The drawing under review shows one solid part. Ordinate dimensions are in mm from its lowest x, y, z. Give positions to 0.01 mm unless a question says otherwise; leave off trailing zeros. Write each loop counter-clockwise with the first axis right and the second up, starting at its lowest first coordinate (ties: lowest second). Pieces come first, ordered by that corner, then holes.
Q1. We need section C-C (x = 4). Write out the cut boundary in (y, z).
Q2. Insertion check: P1, Ø1.7, axis at x = 36.5, z = 17, coming from the +Y side; P2, Ø1.8, axis at y = 2.5, z = 26, coming from the +X side. Each pin has a flat end and moves straight along its axis. Give the tip position at first contact, or say it passes through.
Q3. We need section B-B (z = 4). Write out the cut boundary in (x, y), then the cut area to 3 significant figures.
Q4. We need section D-D (y = 2.5). Give the number of separate pieces and of enclosed holes in the cut face, then the cut area to 3 significant figures.
Q5. For line 1 (X direction, y = 2.05, z = 4); line 2 (Z direction, x = 20.5, y = 4.4); line 3 (X direction, y = 0.55, z = 30.5), list the stretches that pass through material, from the lowest coordinate up.
Q6. We need section A-A (x = 26). Write out the cut boundary in (y, z).
Q7. Mouldability with a two-part tool opening along Z and no side actions: class the marked faces 1, 2 and 3 as released by +Z, released by -Z, zero draft, split by the parting line, or undercut.
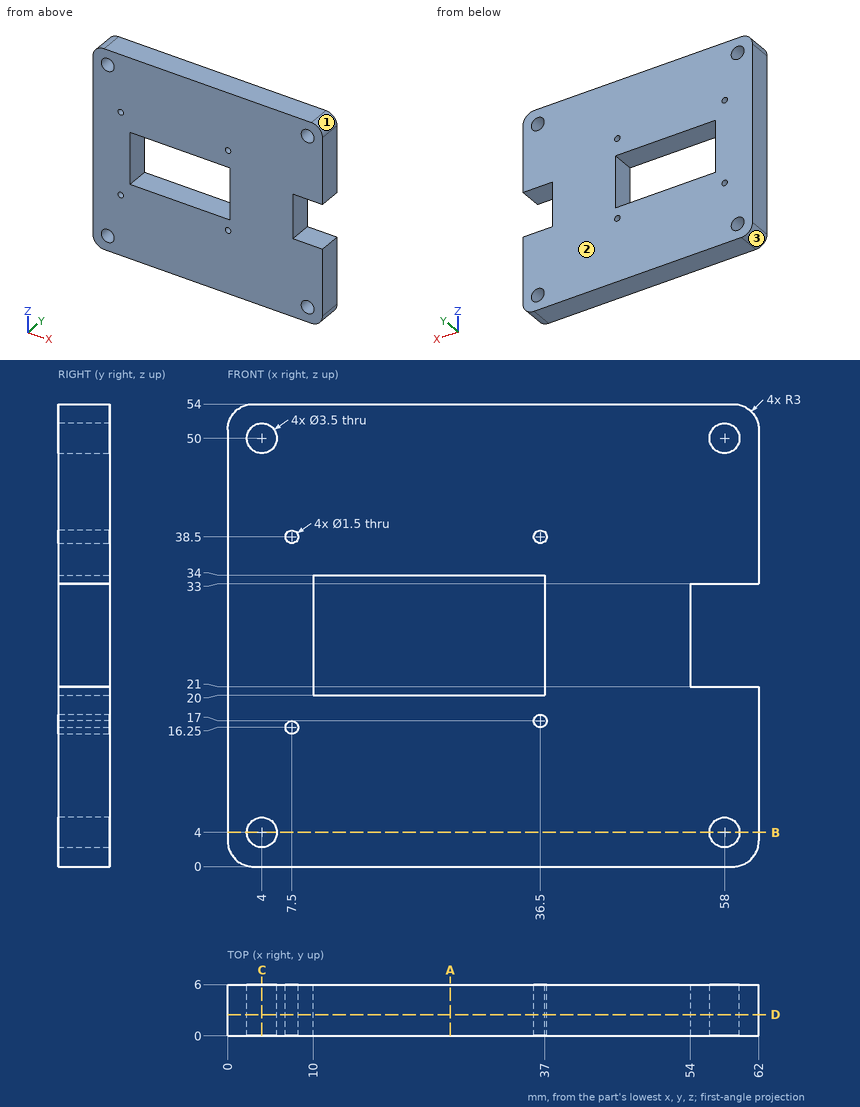
Computed:
1. outline: (0, 0) - (6, 0) - (6, 2.25) - (0, 2.25) - close; (0, 5.75) - (6, 5.75) - (6, 48.25) - (0, 48.25) - close; (0, 51.75) - (6, 51.75) - (6, 54) - (0, 54) - close
2. P1: stops at y = 6
2. P2: stops at x = 54
3. outline: (0, 0) - (2.25, 0) - (2.25, 6) - (0, 6) - close; (5.75, 0) - (56.25, 0) - (56.25, 6) - (5.75, 6) - close; (59.75, 0) - (62, 0) - (62, 6) - (59.75, 6) - close
3. area: 330 mm2
4. separate pieces: 1
4. enclosed holes: 9
4. area: 2,820 mm2
5. line 1: x = 0 to 2.25, 5.75 to 56.25, 59.75 to 62
5. line 2: z = 0 to 20, 34 to 54
5. line 3: x = 0 to 10, 37 to 54
6. outline: (0, 0) - (6, 0) - (6, 20) - (0, 20) - close; (0, 34) - (6, 34) - (6, 54) - (0, 54) - close
7. face 1: released by +Z
7. face 2: zero draft
7. face 3: released by -Z
